Geometry check sheet. Reference: the model listing, model coordinates, mm. Give positions to 0.01 mm unless a question says otherwise; leave off trailing zeros. Order: outer loops, then holes, each group sorted by start corner. A loop starts at its lowest first (then second) coordinate and runs counter-clockwise, first axis right, second up. Notation, with made-up numbers: M 56,-25 L 108,-25 A25 cw 108,7 Z; hole C 24,35.25 d1. An arc over 180 degrees is marked long. Answer as CSV lines item,"result".
from build123d import *

# Parameters (mm, degrees)
SKETCH3_R           = 2
BOSS_EXTRUDE3_DEPTH = 3


with BuildPart() as part:
    # Sketch3 → Boss-Extrude3 (new body)
    with BuildSketch(Plane(origin=(0, 0, 0), x_dir=(1, 0, 0), z_dir=(0, 1, 0))):
        with BuildLine():
            Line((-49.171013104, 56.877731278), (50.828986896, 56.877731278))
            ThreePointArc((50.828986896, 56.877731278), (65.565194963, 70.579032512), (70.828986896, 90))
            Line((70.828986896, 90), (85, 90))
            ThreePointArc((85, 90), (113.045378517, 0), (85, -90))
            Line((85, -90), (70.825442188, -90))
            ThreePointArc((70.825442188, -90), (65.296898803, -71.164130385), (50.828986896, -57.896338511))
            Line((50.828986896, -57.896338511), (-49.171013104, -57.896338511))
            ThreePointArc((-49.171013104, -57.896338511), (-53.39689903, -63.623937963), (-54.893799534, -70.582586985))
            Line((-54.893799534, -70.582586985), (-72.612335341, -70.582586985))
            ThreePointArc((-72.612335341, -70.582586985), (-95.56056104, -38.735568001), (-104.48280247, -0.509303616))
            ThreePointArc((-104.48280247, -0.509303616), (-95.643665217, 37.952810082), (-72.612335341, 70))
            Line((-72.612335341, 70), (-54.893799534, 70))
            ThreePointArc((-54.893799534, 70), (-53.400865269, 62.84206348), (-49.171013104, 56.877731278))
        make_face()
        with Locations((33.401757754, -27.820969354)):
            Circle(SKETCH3_R, mode=Mode.SUBTRACT)
        with Locations((33.401757754, 28.179030646)):
            Circle(SKETCH3_R, mode=Mode.SUBTRACT)
        with Locations((-66.171013104, 43.490696384)):
            Circle(SKETCH3_R, mode=Mode.SUBTRACT)
        with Locations((67.828986896, 43.490696384)):
            Circle(SKETCH3_R, mode=Mode.SUBTRACT)
        with Locations((67.828986896, -44.509303616)):
            Circle(SKETCH3_R, mode=Mode.SUBTRACT)
        with Locations((-66.171013104, -44.509303616)):
            Circle(SKETCH3_R, mode=Mode.SUBTRACT)
    extrude(amount=BOSS_EXTRUDE3_DEPTH)


solid = part.part
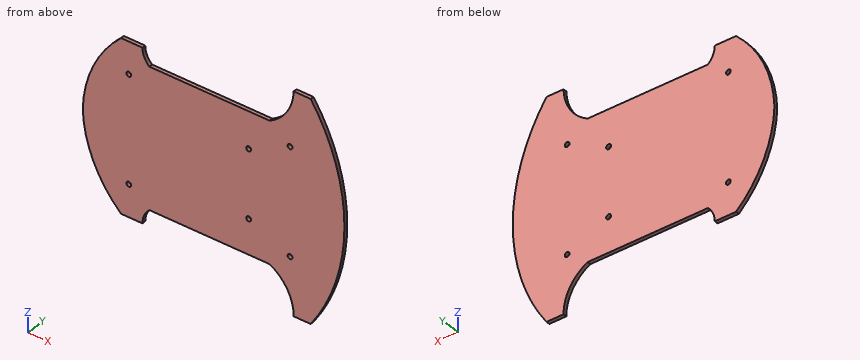
(1) Section check B-B on x = -26. Enter the section's corners in (y, z).
The answers:
outline,"M 0,-56.88 L 3,-56.88 L 3,57.9 L 0,57.9 Z"
(2) Material ranges on line 1 (Z direction, x = -66, y = 1.3); line 2 (Z direction, x = 35, y = 2.7); line 3 (X direction, y = 0.5, z = 45), recorded low to high.
The answers:
line 1,"z = -70 to -45.48, -41.5 to 42.52, 46.5 to 70.58"
line 2,"z = -56.88 to -29.38, -26.98 to 26.62, 29.02 to 57.9"
line 3,"x = -92.44 to -68.11, -64.23 to 65.89, 69.77 to 106.52"
(3) Section check A-A on y = 0.6. Enter the section's corners in (x, z).
The answers:
outline,"M -104.48,0.51 A100 ccw -72.61,-70 L -54.89,-70 A17.91 cw -49.17,-56.88 L 50.83,-56.88 A36.59 cw 70.83,-90 L 85,-90 A158.43 ccw 85,90 L 70.83,90 A36.59 cw 50.83,57.9 L -49.17,57.9 A16.92 cw -54.89,70.58 L -72.61,70.58 A100 ccw Z; hole C -66.17,-43.49 d4; hole C -66.17,44.51 d4; hole C 33.4,-28.18 d4; hole C 33.4,27.82 d4; hole C 67.83,-43.49 d4; hole C 67.83,44.51 d4"
(4) Gauge pin test, flat ends, axial feed: P1, Ø3, axis at x = 67.83, z = 44.51, coming from the -Y side; P2, Ø1.5, axis at x = -10.5, y = 1.5, coming from the +Z side. Record the tip position at first contact, or that the pin passes through.
The answers:
P1,"passes through"
P2,"stops at z = 57.9"
(5) Section check C-C on z = 50. Enter the section's corners in (x, y), then the cut area to 3 significant figures.
The answers:
outline,"M -89.54,0 L 104.95,0 L 104.95,3 L -89.54,3 Z"
area,"583 mm2"
